Geometry: final body of the model. Coordinates: model frame, mm. Face numbers are marked on the shaded views. A direction names the side the tool comes from. Coordinates: 2 decimals unless noted, no trailing zeros. Order: outer loops, then holes, each group sorted by start corner. A loop starts at its lowest first (then second) coordinate and runs counter-clockwise, first axis right, second up. Notation, with made-up numbers: M -1,25 L 48,25 A23 ccw 48,39 Z; hole C 37,52.5 d3. An arc over 180 degrees is marked long. Use CSV: the item, a comma, the result in double quotes. Start each with the question number.
1. First-contact query: P1, Ø5, axis at x = 0, y = 0, coming from the +Z side; P2, Ø2, axis at x = 3, z = 0.5, coming from the +Y side; P3, Ø3, axis at y = -8.5, z = 1.5, coming from the +X side; P4, Ø6, axis at x = -7.5, y = 8.5, coming from the +Z side. Flat tips, straight axial feed; report the tip coordinate or a pass-through.
2. Pull-direction query (Y, two-part tool) for the marked faces 1, 2 and 3; classes: pulls with the +Y half, pulls with the -Y half, needs draft (parallel to the pull), parting line crosses it, or undercut.
3. Material intervals for line 1 (Y direction, x = 0, z = -1.5); line 2 (Y direction, x = 0, z = 3.55) (3 decimals); line 3 (Z direction, x = 8.5, y = -5.75), sorted ascending.
4. Set-up query: the marked faces 4, 5 and 6. Return all of +Z, -Z, +X, -X, +Y, -Y with unobstructed straight access to the full face (end or side cutting, diameter ignored); none if empty.
5. Section query A-A on z = 0.5. Return the cut outline in (x, y), and give its area (3 significant figures).
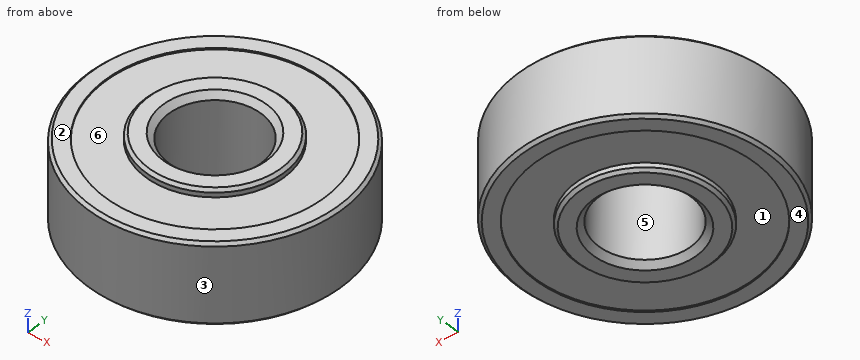
from build123d import *

# Parameters (mm, degrees)
SKETCH1_R           = 11
SKETCH1_R_2         = 9.5
BOSS_EXTRUDE1_DEPTH = 3.5
SKETCH1_4_R         = 6
SKETCH1_4_R_2       = 4
BOSS_EXTRUDE2_DEPTH = 4.025
SKETCH1_5_R         = 9.5
SKETCH1_5_R_2       = 6
BOSS_EXTRUDE3_DEPTH = 3.375
CHAMFER1_SIZE       = 0.5
CHAMFER2_SIZE       = 0.25


with BuildPart() as part:
    # Sketch1 → Boss-Extrude1 (new body, symmetric)
    with BuildSketch(Plane.XY):
        Circle(SKETCH1_R)
        Circle(SKETCH1_R_2, mode=Mode.SUBTRACT)
    extrude(amount=BOSS_EXTRUDE1_DEPTH, both=True)



with BuildPart() as body_2:
    # Sketch1<4> → Boss-Extrude2 (new body, symmetric)
    with BuildSketch(Plane.XY):
        Circle(SKETCH1_4_R)
        Circle(SKETCH1_4_R_2, mode=Mode.SUBTRACT)
    extrude(amount=BOSS_EXTRUDE2_DEPTH, both=True)


with BuildPart() as part_1:
    add(part.part)

    add(body_2.part)  # Boss-Extrude3 merges body 2
    # Sketch1<5> → Boss-Extrude3 (add, symmetric)
    with BuildSketch(Plane.XY):
        Circle(SKETCH1_5_R)
        Circle(SKETCH1_5_R_2, mode=Mode.SUBTRACT)
    extrude(amount=BOSS_EXTRUDE3_DEPTH, both=True)

    # Chamfer1
    chamfer1_edges = [part_1.edges().sort_by_distance(p)[0] for p in [
        (-4, 0, 4.025),
        (-4, 0, -4.025),
    ]]
    chamfer(chamfer1_edges, length=CHAMFER1_SIZE)

    # Chamfer2
    chamfer2_edges = [part_1.edges().sort_by_distance(p)[0] for p in [
        (-11, 0, 3.5),
        (-6, 0, -4.025),
        (-6, 0, 4.025),
        (-11, 0, -3.5),
    ]]
    chamfer(chamfer2_edges, length=CHAMFER2_SIZE)


solid = part_1.part
Results list:
1,P1,"passes through"
1,P2,"stops at y = 10.82"
1,P3,"stops at x = 8.49"
1,P4,"stops at z = 3.5"
2,face 1,"undercut"
2,face 2,"needs draft"
2,face 3,"parting line crosses it"
3,line 1,"y = -11 to -4, 4 to 11"
3,line 2,"y = -6 to -4.025, 4.025 to 6"
3,line 3,"z = -3.5 to 3.5"
4,face 4,"-Z"
4,face 5,"+Z, -Z"
4,face 6,"+Z"
5,outline,"C 0,0 d22; hole C 0,0 d8"
5,area,"330 mm²"
